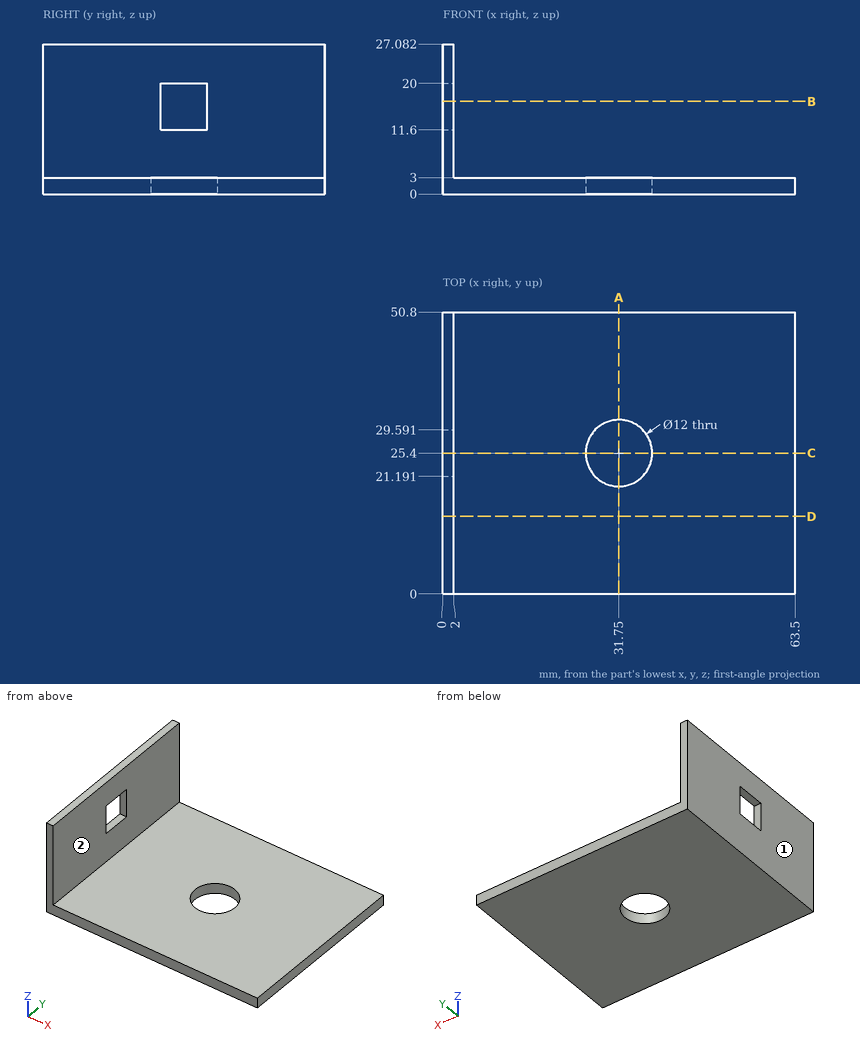
Input: dimensioned drawing with shaded views. Units: mm. Origin: part minimum x, y, z. A direction names the side the tool comes from. Round coordinates to 2 decimals unless told otherwise and drop trailing zeros. Loops run counter-clockwise (first coordinate to the right, second up) from the corner with the lowest first, then second, coordinate; pieces in that order, holes last. Notation, with made-up numbers: (28, 25.5) -> (49, 25.5) arc R21 ccw to (49, 63.5) -> close; hole circle Ø1 at (-14, 23.5). An arc over 180 degrees is marked (long way). Answer as a JSON object with one key per item and string values. Group by question number.
1) Section query D-D on y = 14. Output: boundary loops of the cut face in (x, z).
2) Section query A-A on x = 31.75. Output: boundary loops of the cut face in (y, z).
3) Section query B-B on z = 16.75. Output: boundary loops of the cut face in (x, y), plus the area to 3 significant figures.
4) Pin query (flat end, axial travel): pin 1 (7 mm diameter, centred on x = 31.75, y = 25.4, fed in from -Z); pin 2 (5 mm diameter, centred on y = 30.5, z = 15, fed in from +X); pin 3 (0.6 mm diameter, centred on x = 1, y = 24, fed in from -Z). Return the tip coordinate at first contact, or that it passes through.
5) Section query C-C on y = 25.4. Output: boundary loops of the cut face in (x, z).
6) Ray query, L1, parallel to Y at x = 31.75, z = 1.1; L2, parallel to Z at x = 52, y = 12; L3, parallel to X at y = 36, z = 9. Return the intervals inside material, ascending.
7) Reachability of the marked faces 1 and 2 from +Z, -Z, +X, -X, +Y, -Y: full face, straight path, thin tool, end or side. Return the list, or none.
Reply:
{
 "1": {"outline": "(0, 0) -> (63.5, 0) -> (63.5, 3) -> (2, 3) -> (2, 27.08) -> (0, 27.08) -> close"},
 "2": {"outline": "(0, 0) -> (19.4, 0) -> (19.4, 3) -> (0, 3) -> close; (31.4, 0) -> (50.8, 0) -> (50.8, 3) -> (31.4, 3) -> close"},
 "3": {"outline": "(0, 0) -> (2, 0) -> (2, 21.19) -> (0, 21.19) -> close; (0, 29.59) -> (2, 29.59) -> (2, 50.8) -> (0, 50.8) -> close", "area": "84.8 mm2"},
 "4": {"pin 1": "passes through", "pin 2": "stops at x = 2", "pin 3": "stops at z = 0"},
 "5": {"outline": "(0, 0) -> (25.75, 0) -> (25.75, 3) -> (2, 3) -> (2, 11.6) -> (0, 11.6) -> close; (0, 20) -> (2, 20) -> (2, 27.08) -> (0, 27.08) -> close; (37.75, 0) -> (63.5, 0) -> (63.5, 3) -> (37.75, 3) -> close"},
 "6": {"L1": "y = 0 to 19.4, 31.4 to 50.8", "L2": "z = 0 to 3", "L3": "x = 0 to 2"},
 "7": {"face 1": "+Z, -Z, -X, +Y, -Y", "face 2": "+Z, +X, +Y, -Y"}
}
